```python
from build123d import *

# Parameters (mm, degrees)
SKETCH1_R               = 15
SKETCH1_R_2             = 13
BOSS_EXTRUDE1_DEPTH     = 282.5
SKETCH3_W               = 10
SKETCH3_H               = 50
CUT_EXTRUDE1_DEPTH      = 282.5
CUT_EXTRUDE2_DEPTH      = 284.29534059
CUT_EXTRUDE2_DEPTH_BACK = 284.29534059
SKETCH4_R               = 4


with BuildPart() as part:
    # Sketch1 → Boss-Extrude1 (new, symmetric)
    with BuildSketch(Plane(origin=(0, 0, 0), x_dir=(1, 0, 0), z_dir=(0, 1, 0))):
        with Locations(Location((0, 0, 0), (0, 0, 270))):
            Circle(SKETCH1_R)
        with Locations(Location((0, 0, 0), (0, 0, 270))):
            Circle(SKETCH1_R_2, mode=Mode.SUBTRACT)
    extrude(amount=BOSS_EXTRUDE1_DEPTH, both=True)

    # Sketch3 → Cut-Extrude1 (cut, symmetric)
    with BuildSketch(Plane(origin=(0, 0, 0), x_dir=(0, 0, -1), z_dir=(1, 0, 0))):
        with Locations((0, -257.5)):
            Rectangle(SKETCH3_W, SKETCH3_H)
    extrude(amount=CUT_EXTRUDE1_DEPTH, both=True, mode=Mode.SUBTRACT)

    # Sketch4 → Cut-Extrude2 (cut, two sides: drawn at the far end of the back side and taken through both)
    with BuildSketch(Plane.XY.offset(-CUT_EXTRUDE2_DEPTH_BACK)):
        with Locations((0, -247.5)):
            Circle(SKETCH4_R)
    extrude(amount=CUT_EXTRUDE2_DEPTH + CUT_EXTRUDE2_DEPTH_BACK, mode=Mode.SUBTRACT)


solid = part.part
```
Geometry check sheet. Reference: the model listing, model coordinates, mm. Round coordinates to 2 decimals unless told otherwise and drop trailing zeros. Order: outer loops, then holes, each group sorted by start corner. A loop starts at its lowest first (then second) coordinate and runs counter-clockwise, first axis right, second up. Notation, with made-up numbers: (31.5, -2.75) - (52.5, -2.75) arc R19 ccw to (52.5, 34.25) - close; hole circle Ø2 at (55, 14). An arc over 180 degrees is marked (long way). Use a Markdown table: item, result. Add a question column.
(1) Sectioned sample at A-A, the plane z = 0. Enter the section's corners in (x, y).
(2) Material ranges on line 1 along Z through (x, y) = (0, 134); line 2 along Y through (x, z) = (0, 14), recorded low to high. Write a range as [from, to].
(3) Release check for a two-part mould opening along Z. For faces 1 (the cylindrical face through (3.9, -4, 12.4)), 2 (the cylindrical face through (-5.745, 3.955, 13.856)), 3 (the flat face through (1.1, -282.5, -13.4)) record: pulls with the +Z half, pulls with the -Z half, needs draft (parallel to the pull), parting line crosses it, or undercut.
(4) Depth check by flat-ended pin: pin 1 (6 mm diameter, centred on y = -73.5, z = 8.5, fed in from -X); pin 2 (1 mm diameter, centred on x = 11, z = 12, fed in from +Y); pin 3 (2 mm diameter, centred on x = -11, y = 52, fed in from +Z); pin 4 (0.9 mm diameter, centred on x = 14, z = 1, fed in from -Y). Enter the tip coordinate at first touch or a pass-through.
(5) Sectioned sample at B-B, the plane y = -85.5. Enter the section's corners in (x, z).
Answers below:
| question | item | result |
|---|---|---|
| 1 | outline | (-15, -232.5) - (-13, -232.5) - (-13, 282.5) - (-15, 282.5) - close; (13, -232.5) - (15, -232.5) - (15, 282.5) - (13, 282.5) - close |
| 2 | line 1 | [-15, -13], [13, 15] |
| 2 | line 2 | [-282.5, -251.5], [-243.5, 282.5] |
| 3 | face 1 | undercut |
| 3 | face 2 | parting line crosses it |
| 3 | face 3 | needs draft |
| 4 | pin 1 | x = -13.96 |
| 4 | pin 2 | through |
| 4 | pin 3 | z = 11.18 |
| 4 | pin 4 | y = -232.5 |
| 5 | outline | circle Ø30 at (0, 0); hole circle Ø26 at (0, 0) |
